Check sheet for the drawn part. Datum: minimum x, y, z corner. Units: mm. A direction names the side the tool comes from. Round coordinates to 2 decimals unless told otherwise and drop trailing zeros. Write each loop counter-clockwise with the first axis right and the second up, starting at its lowest first coordinate (ties: lowest second). Pieces come first, ordered by that corner, then holes. Notation, with made-up numbers: M 89.25,-25.75 L 100.25,-25.75 A17 cw 100.25,-5.75 Z; hole C -4,66 d5. An arc over 180 degrees is marked long. One line per item, written item: value. Start each with the question number.
1. Depth check by flat-ended pin: P1, Ø6, axis at x = 22.5, z = 24.5, coming from the -Y side. Enter the tip coordinate at first touch or a pass-through.
2. Section check A-A (y = 7.62). Record the boundary of the cut face in (x, z) (1 decimal).
3. Section check D-D (x = 16.5). Record the boundary of the cut face in (y, z) (1 decimal).
4. Section check C-C (x = 23.5). Record the boundary of the cut face in (y, z).
5. Section check B-B (z = 36.5). Record the boundary of the cut face in (x, y).
6. Release check for a two-part mould opening along Z. For the marked faces 3, 4, 5 and 6 record: pulls with the +Z half, pulls with the -Z half, needs draft (parallel to the pull), parting line crosses it, or undercut.
7. Access from +Z, -Z, +X, -X, +Y, -Y to the whole of each face (thin tool, end or side, straight path). Record for the marked faces 1 and 2.
8. Scan lines: probe 1 along Z at (x, y) = (2.5, 3); probe 2 along X at (y, z) = (7.62, 64.05) (1 decimal); probe 3 along X at (y, z) = (1.75, 61). Record each from-to range of solid material in increasing order. Write a range as [from, to].
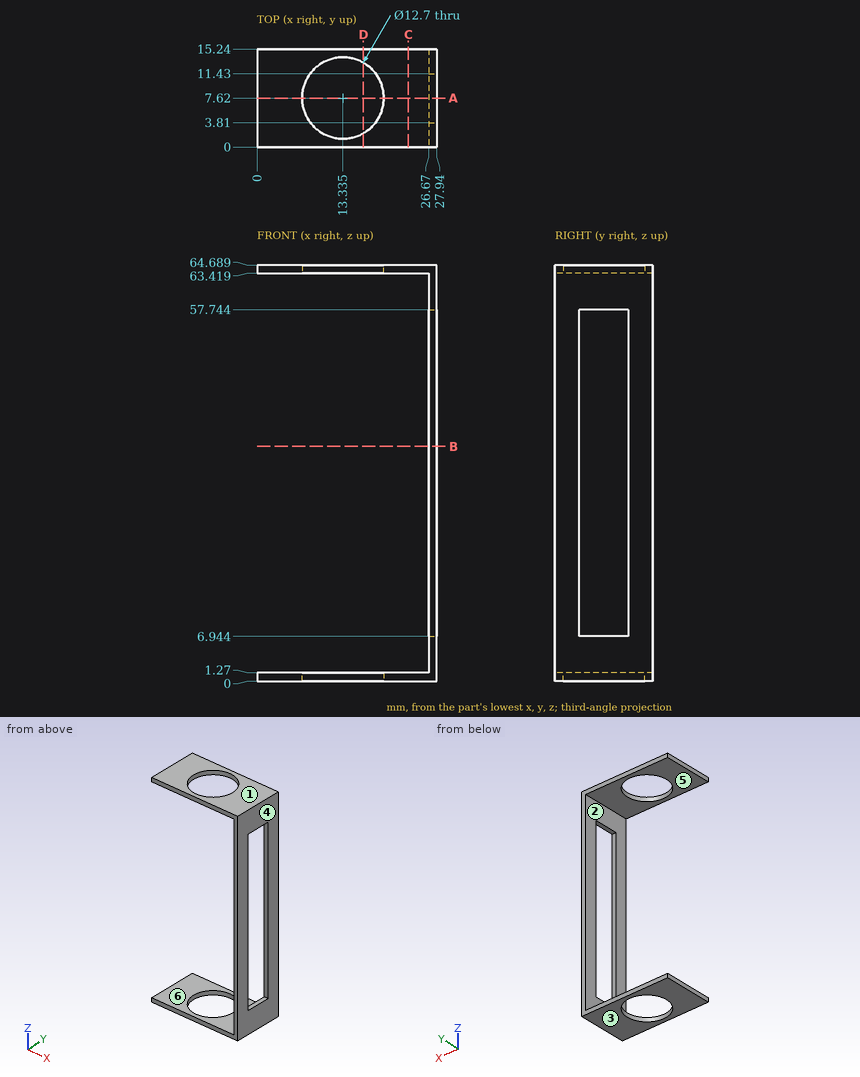
Result sheet:
1. P1: passes through
2. outline: M 0,0 L 7,0 L 7,1.3 L 0,1.3 Z; M 0,63.4 L 7,63.4 L 7,64.7 L 0,64.7 Z; M 19.7,0 L 27.9,0 L 27.9,6.9 L 26.7,6.9 L 26.7,1.3 L 19.7,1.3 Z; M 19.7,63.4 L 26.7,63.4 L 26.7,57.7 L 27.9,57.7 L 27.9,64.7 L 19.7,64.7 Z
3. outline: M 0,0 L 2.1,0 L 2.1,1.3 L 0,1.3 Z; M 0,63.4 L 2.1,63.4 L 2.1,64.7 L 0,64.7 Z; M 13.1,0 L 15.2,0 L 15.2,1.3 L 13.1,1.3 Z; M 13.1,63.4 L 15.2,63.4 L 15.2,64.7 L 13.1,64.7 Z
4. outline: M 0,0 L 15.24,0 L 15.24,1.27 L 0,1.27 Z; M 0,63.42 L 15.24,63.42 L 15.24,64.69 L 0,64.69 Z
5. outline: M 26.67,0 L 27.94,0 L 27.94,3.81 L 26.67,3.81 Z; M 26.67,11.43 L 27.94,11.43 L 27.94,15.24 L 26.67,15.24 Z
6. face 3: pulls with the -Z half
6. face 4: needs draft
6. face 5: undercut
6. face 6: undercut
7. face 1: +Z, +X, -X, +Y, -Y
7. face 2: -X, +Y, -Y
8. probe 1: z = [0, 1.27], [63.42, 64.69]
8. probe 2: x = [0, 7], [19.7, 27.9]
8. probe 3: x = [26.67, 27.94]
